```python
from build123d import *

# Parameters (mm, degrees)
F1_DEPTH = 447.675
F2_R     = 19.05
F3_DEPTH = 25.4


with BuildPart() as f1:
    # F0 (on Front) → F1 (new body)
    with BuildSketch(Plane.XZ):
        with BuildLine():
            Line((113.057586, 185.428598), (3.12076, 185.428598))
            Line((3.12076, 185.428598), (-106.816067, 185.428598))
            ThreePointArc((-106.816067, 185.428598), (-120.143025, 179.990897), (-125.861793, 166.782109))
            Line((-125.861793, 166.782109), (-133.40424, -189.221402))
            Line((-133.40424, -189.221402), (3.12076, -189.221402))
            Line((3.12076, -189.221402), (139.64576, -189.221402))
            Line((139.64576, -189.221402), (132.103312, 166.782109))
            ThreePointArc((132.103312, 166.782109), (126.384544, 179.990897), (113.057586, 185.428598))
        make_face()
    extrude(amount=-F1_DEPTH)

    # F2 (on face) → F3 (join)
    with BuildSketch(Plane.XZ):
        with Locations((70.142567, 78.941181)):
            Circle(F2_R)
        with Locations((70.142567, -6.655197)):
            Circle(F2_R)
    extrude(amount=F3_DEPTH)


solid = f1.part
```
The listing builds one solid part. Answer for the finished solid, in the listing's coordinates (mm). A direction names the side the tool comes from. Round coordinates to 2 decimals unless told otherwise and drop trailing zeros. Write each loop counter-clockwise with the first axis right and the second up, starting at its lowest first coordinate (ties: lowest second). Pieces come first, ordered by that corner, then holes. Notation, with made-up numbers: (34, -2) -> (75, -2) arc R15 cw to (75, 10) -> close; hole circle Ø1 at (63, -21.75). An arc over 180 degrees is marked (long way). Answer as a JSON object with one key per item and string values. Group by question number.
Q1. Section B-B (z = -12.5) is taken. Write down the section's boundary in (x, y) (3 decimals), plus the area to 3 significant figures.
Q2. Straight lines are drawn through the part: line 1 along Y through (x, z) = (-82, -169.5) (3 decimals); line 2 along X through (y, z) = (248.5, -75); line 3 along X through (y, z) = (6, 133.5). For each, find the intervals that lie inside material, in ascending order.
Q3. Section D-D (z = -113) is taken. Write down the section's boundary in (x, y) (3 decimals).
Q4. Each of these flat-tipped pins is pushed along its axis until it touches: pin 1 Ø2 at (y, z) = (286.5, 40) entering from +X; pin 2 Ø1.5 at (x, z) = (-4, 96) entering from -Y; pin 3 Ø3 at (y, z) = (259.5, 86) entering from +X. Where does it stop, or does it pass through?
Q5. Section A-A (y = 35) is taken. Write down the section's boundary in (x, z).
Q6. Which of the six approach directions +Z, -Z, +X, -X, +Y, -Y give full straight-line access (tool end or side, diameter ignored) to faces 1 (the face through (51.11, -12.52, -5.82)), 2 (the face through (126.531, 220.704, 179.846))?
Q7. Determine the mould class of faces 3 (the face through (70, -25.4, 79)), 4 (the face through (55.025, -12.522, 67.35)), 5 (the face through (5, 221, 185.429)) for opening direction Z: pulls with the +Z half, pulls with the -Z half, needs draft (parallel to the pull), parting line crosses it, or undercut.
Q8. Section C-C (x = 1) is taken. Write down the section's boundary in (y, z) (3 decimals).
Check values:
{
 "1": {"outline": "(-129.66, 0) -> (52.011, 0) -> (52.011, -25.4) -> (88.274, -25.4) -> (88.274, 0) -> (135.902, 0) -> (135.902, 447.675) -> (-129.66, 447.675) -> close", "area": "120,000 mm^2"},
 "2": {"line 1": "0 to 447.675", "line 2": "-130.98 to 137.23", "line 3": "-126.57 to 132.81"},
 "3": {"outline": "(-131.789, 0) -> (138.031, 0) -> (138.031, 447.675) -> (-131.789, 447.675) -> close"},
 "4": {"pin 1": "x = 134.81", "pin 2": "y = 0", "pin 3": "x = 133.85"},
 "5": {"outline": "(-133.4, -189.22) -> (139.65, -189.22) -> (132.1, 166.78) arc R19.05 ccw to (113.06, 185.43) -> (-106.82, 185.43) arc R19.05 ccw to (-125.86, 166.78) -> close"},
 "6": {"face 1": "-Y", "face 2": "+Z, +X, +Y, -Y"},
 "7": {"face 3": "needs draft", "face 4": "undercut", "face 5": "pulls with the +Z half"},
 "8": {"outline": "(0, -189.221) -> (447.675, -189.221) -> (447.675, 185.429) -> (0, 185.429) -> close"}
}
